Can you work these out from the drawing? Everything is in mm from the part's minimum corner. A direction names the side the tool comes from. Coordinates: 2 decimals unless noted, no trailing zeros. Loops run counter-clockwise (first coordinate to the right, second up) from the corner with the lowest first, then second, coordinate; pieces in that order, holes last. Notation, with made-up numbers: M 67.25,-35 L 78.25,-35 A20 cw 78.25,-14 Z; hole C -10,65 d8. An arc over 180 degrees is marked long. Use CSV: the item, a comma, the result in double quotes. Start each with the question number.
Q1. If we section it at A-A (z = 6.35): Please give me the cut outline in (x, y) (3 decimals), and give its area (3 significant figures).
Q2. Which directions (+Z, -Z, +X, -X, +Y, -Y) give clear straight access to the entire face, cutting with the end or side of a thin tool? Please do the marked faces 1, 2 and 3.
Q3. Please list where these lines run through material, in increasing order: probe 1 along Y at (x, z) = (3, 9.75); probe 2 along Z at (x, y) = (6.25, 40); probe 3 along Z at (x, y) = (8.5, 34.5). Write a range as [from, to].
Q4. For pin 1 Ø5 at (x, z) = (10.5, 11.5) entering from +Y; pin 2 Ø3 at (y, z) = (28.5, 3.5) entering from +X; pin 3 Ø6 at (x, y) = (4.5, 19) entering from +Z (3 decimals), each with a flat end and sliding along its axis, tell me the tip position at first contact or that it passes through.
Q5. If we section it at C-C (y = 46.5): Please give me the cut outline in (x, z) (3 decimals).
Q6. If we section it at B-B (x = 6.35): Please give me the cut outline in (y, z) (3 decimals).
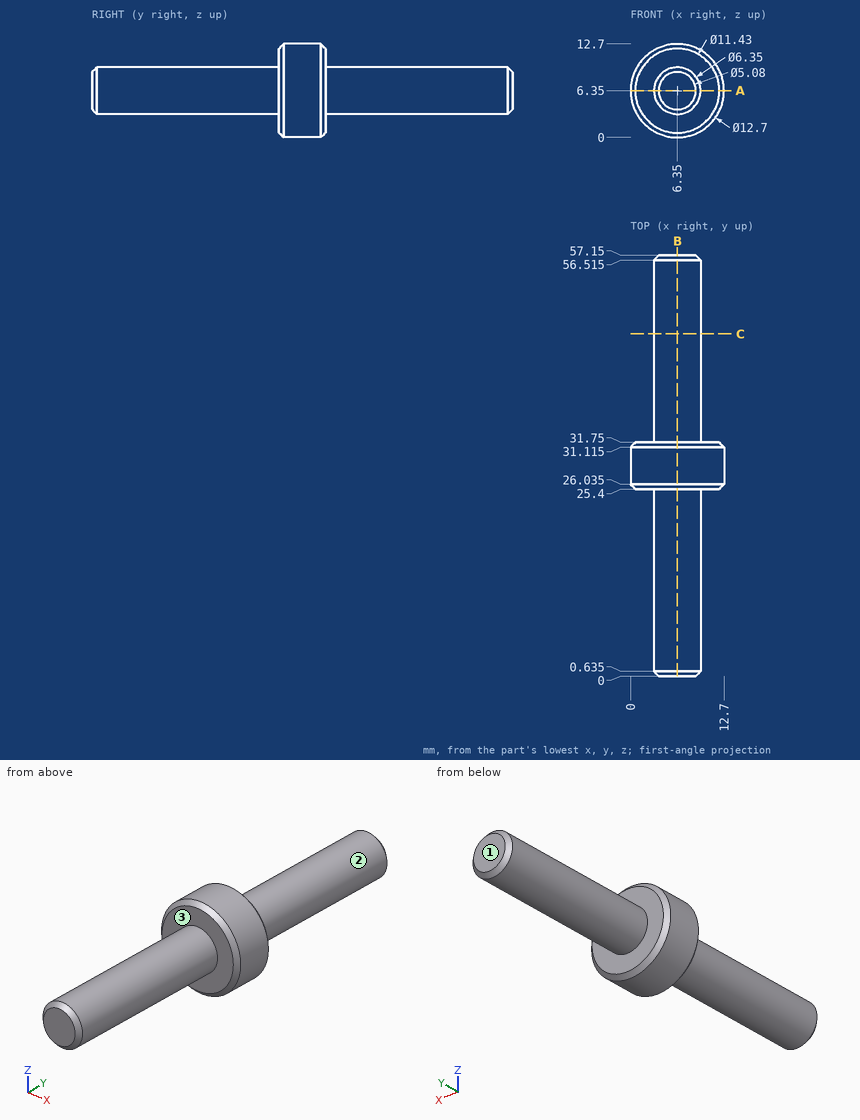
Results below:
1,outline,"M 0,26.035 L 0.635,25.4 L 3.175,25.4 L 3.175,0.635 L 3.81,0 L 8.89,0 L 9.525,0.635 L 9.525,25.4 L 12.065,25.4 L 12.7,26.035 L 12.7,31.115 L 12.065,31.75 L 9.525,31.75 L 9.525,56.515 L 8.89,57.15 L 3.81,57.15 L 3.175,56.515 L 3.175,31.75 L 0.635,31.75 L 0,31.115 Z"
1,area,"402 mm^2"
2,face 1,"+Z, -Z, +X, -X, +Y"
2,face 2,"+Y"
2,face 3,"-Y"
3,probe 1,"[25.4, 31.75]"
3,probe 2,"[3.18, 9.52]"
3,probe 3,"[4.01, 8.69]"
4,pin 1,"y = 31.75"
4,pin 2,"x = 12.55"
4,pin 3,"z = 9.525"
5,outline,"C 6.35,6.35 d6.35"
6,outline,"M 0,3.81 L 0.635,3.175 L 25.4,3.175 L 25.4,0.635 L 26.035,0 L 31.115,0 L 31.75,0.635 L 31.75,3.175 L 56.515,3.175 L 57.15,3.81 L 57.15,8.89 L 56.515,9.525 L 31.75,9.525 L 31.75,12.065 L 31.115,12.7 L 26.035,12.7 L 25.4,12.065 L 25.4,9.525 L 0.635,9.525 L 0,8.89 Z"
